The figure shows three views and two pictorial views of one solid part (mm, origin at its lowest corner). Answer the questions. A direction names the side the tool comes from. Coordinates: 2 decimals unless noted, no trailing zeros. Order: outer loops, then holes, each group sorted by start corner. A loop starts at its lowest first (then second) coordinate and runs counter-clockwise, first axis right, second up. Notation, with made-up numbers: M -38,56 L 17,56 A25 cw 17,82 Z; hole C 47,73.5 d8. An arc over 180 degrees is marked long. Answer in a Markdown table with one row per item. Add a question column.
Item 1: The part is cut by section A-A (x = 18.75). Write down the section's boundary in (y, z).
Item 2: Consider line 1 (Z direction, x = 23, y = 2); line 2 (Y direction, x = 9.5, z = 1.75); line 3 (X direction, y = 11.5, z = 4.25). Determine where each line is inside the solid, lowest interval first. Write a range as from..to.
Item 3: Flat-ended cylindrical pins translate along their axes: pin 1 Ø3 at (y, z) = (10.5, 5) entering from +X; pin 2 Ø1 at (y, z) = (11.5, 4.5) entering from -X; pin 3 Ø7.5 at (x, y) = (16, 7.5) entering from -Z. Find the tip coordinate at first contact, or state that the pin passes through.
Item 4: The part is cut by section C-C (y = 12.25). Write down the section's boundary in (x, z).
Item 5: The part is cut by section D-D (z = 7.5). Write down the section's boundary in (x, y).
Item 6: Which of the six approach directions +Z, -Z, +X, -X, +Y, -Y give full straight-line access (tool end or side, diameter ignored) to the marked faces 1, 2, 3, 4 and 5?
Item 7: The part is cut by section B-B (z = 2.5). Write down the section's boundary in (x, y), then the cut area to 3 significant figures.
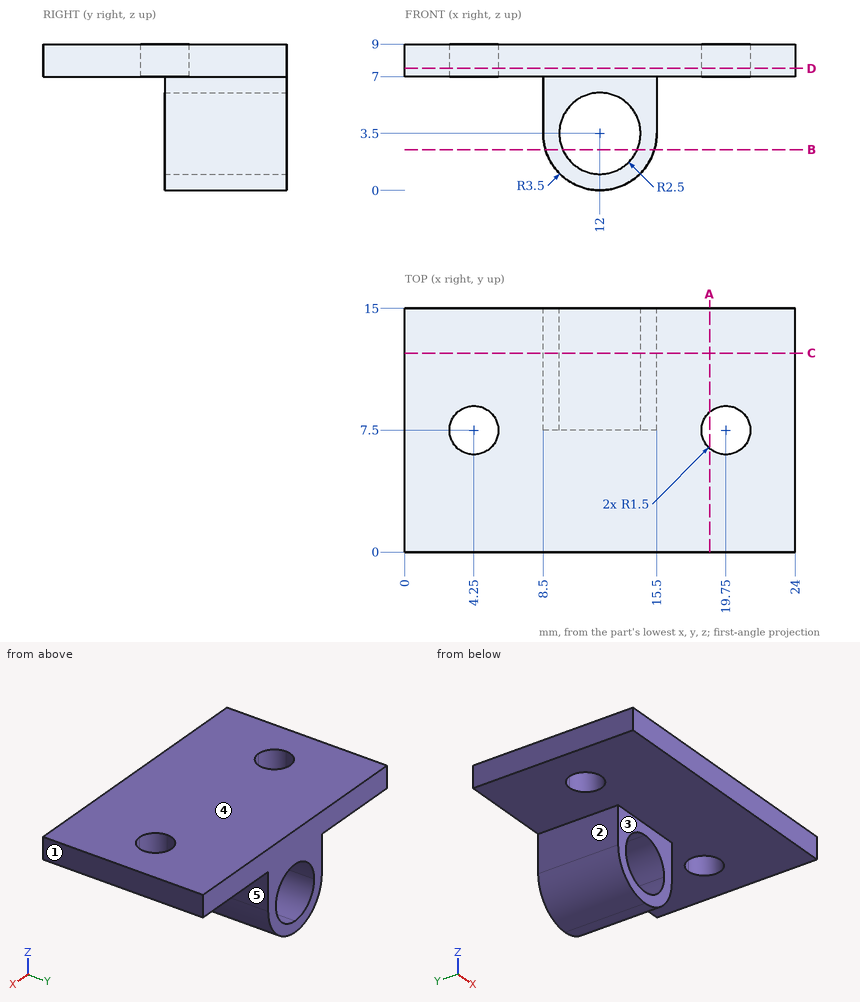
Reply:
| question | item | result |
|---|---|---|
| 1 | outline | M 0,7 L 6.38,7 L 6.38,9 L 0,9 Z; M 8.62,7 L 15,7 L 15,9 L 8.62,9 Z |
| 2 | line 1 | z = 7..9 |
| 2 | line 2 | y = 7.5..15 |
| 2 | line 3 | x = 8.5..9.62, 14.38..15.5 |
| 3 | pin 1 | stops at x = 15.5 |
| 3 | pin 2 | stops at x = 8.5 |
| 3 | pin 3 | stops at z = 0.01 |
| 4 | outline | M 0,7 L 8.5,7 L 8.5,3.5 A3.5 ccw 15.5,3.5 L 15.5,7 L 24,7 L 24,9 L 0,9 Z; hole C 12,3.5 d5 |
| 5 | outline | M 0,0 L 24,0 L 24,15 L 0,15 Z; hole C 4.25,7.5 d3; hole C 19.75,7.5 d3 |
| 6 | face 1 | +Z, -Z, +X, +Y, -Y |
| 6 | face 2 | -Z, -X, +Y, -Y |
| 6 | face 3 | -Z, +X, -X, -Y |
| 6 | face 4 | +Z, +X, -X, +Y, -Y |
| 6 | face 5 | -Z, +X, +Y, -Y |
| 7 | outline | M 8.65,7.5 L 9.71,7.5 L 9.71,15 L 8.65,15 Z; M 14.29,7.5 L 15.35,7.5 L 15.35,15 L 14.29,15 Z |
| 7 | area | 15.9 mm2 |
